```python
from build123d import *

# Parameters (mm, degrees)
SKETCH1_R              = 21.209
EXTRUDE1_DEPTH         = 63.5
SKETCH2_R              = 17.78
EXTRUDE2_DEPTH         = 25.4
EXTRUDE2_DRAFT         = -2.87
CIRPATTERN1_COUNT      = 12
CHAMFER2_SIZE          = 0.254
CHAMFER2_SIZE2         = 0.267741651
CHAMFER2_EDGE_2_SIZE   = 0.254
CHAMFER2_EDGE_2_SIZE2  = 0.267741651
CHAMFER2_EDGE_3_SIZE   = 0.254
CHAMFER2_EDGE_3_SIZE2  = 0.267741651
CHAMFER2_EDGE_4_SIZE   = 0.254
CHAMFER2_EDGE_4_SIZE2  = 0.267741651
CHAMFER2_EDGE_5_SIZE   = 0.254
CHAMFER2_EDGE_5_SIZE2  = 0.267741651
CHAMFER2_EDGE_6_SIZE   = 0.254
CHAMFER2_EDGE_6_SIZE2  = 0.267741651
CHAMFER2_EDGE_7_SIZE   = 0.254
CHAMFER2_EDGE_7_SIZE2  = 0.267741651
CHAMFER2_EDGE_8_SIZE   = 0.254
CHAMFER2_EDGE_8_SIZE2  = 0.267741651
CHAMFER2_EDGE_9_SIZE   = 0.254
CHAMFER2_EDGE_9_SIZE2  = 0.267741651
CHAMFER2_EDGE_10_SIZE  = 0.254
CHAMFER2_EDGE_10_SIZE2 = 0.267741651
CHAMFER2_EDGE_11_SIZE  = 0.254
CHAMFER2_EDGE_11_SIZE2 = 0.267741651
CHAMFER2_EDGE_12_SIZE  = 0.254
CHAMFER2_EDGE_12_SIZE2 = 0.267741651


with BuildPart() as part:
    # Sketch1 → Extrude1 (new body)
    with BuildSketch(Plane(origin=(0, 0, 0), x_dir=(0, 0, -1), z_dir=(1, 0, 0))):
        Circle(SKETCH1_R)
    extrude(amount=EXTRUDE1_DEPTH)


with BuildPart() as extrude2_tool:
    # Sketch2 → Extrude2 (with draft: the straight prism first)
    with BuildSketch(Plane(origin=(63.5, 0, 0), x_dir=(0, 0, -1), z_dir=(1, 0, 0))):
        Circle(SKETCH2_R)
    extrude(amount=-EXTRUDE2_DEPTH)
    # Extrude2: the draft: its side faces are tilted about the plane it starts from
    extrude2_sides = [extrude2_tool.faces().sort_by_distance(p)[0] for p in [
        (50.8, 0, 17.78),
    ]]
    draft(extrude2_sides, Plane(origin=(63.5, 0, 0), x_dir=(0, 0, -1), z_dir=(1, 0, 0)), EXTRUDE2_DRAFT)


with BuildPart() as part_1:
    add(part.part)

    # Extrude2: cut by extrude2_tool
    add(extrude2_tool.part, mode=Mode.SUBTRACT)

    # Sketch4 → 3/16 (0.1875) Diameter Hole1 (revolve, cut)
    with BuildSketch(Plane(origin=(63.5, 0, 16.51), x_dir=(0, 0, -1), z_dir=(0, 1, 0))):
        Polygon((0, 0), (0, 33.180799349), (2.38125, 31.75), (2.38125, 0), align=None)
    f_3_16_0_1875_diameter_hole1 = revolve(axis=Axis((69.85, 0, 16.51), (-1, 0, 0)), mode=Mode.SUBTRACT)

    # CirPattern1: 3/16 (0.1875) Diameter Hole1 ×12 about axis
    cirpattern1_axis = Axis((0, 0, 0), (1, 0, 0))
    for i in range(1, CIRPATTERN1_COUNT):
        add(f_3_16_0_1875_diameter_hole1.rotate(cirpattern1_axis, i * 360 / CIRPATTERN1_COUNT), mode=Mode.SUBTRACT)

    # Chamfer2
    chamfer2_edges = [part_1.edges().sort_by_distance(p)[0] for p in [
        (63.5, 17.174161191, -4.601802622),
    ]]
    chamfer2_side = [part_1.faces().sort_by_distance(p)[0] for p in [
        (63.5, 0, 20.609118891),
    ]]
    chamfer(chamfer2_edges, length=CHAMFER2_SIZE, length2=CHAMFER2_SIZE2, reference=chamfer2_side[0])

    # Chamfer2 edge 2
    chamfer2_edge_2_edges = [part_1.edges().sort_by_distance(p)[0] for p in [
        (63.5, 12.572358569, -12.572358569),
    ]]
    chamfer2_edge_2_side = [part_1.faces().sort_by_distance(p)[0] for p in [
        (63.5, 0, 20.609118891),
    ]]
    chamfer(chamfer2_edge_2_edges, length=CHAMFER2_EDGE_2_SIZE, length2=CHAMFER2_EDGE_2_SIZE2, reference=chamfer2_edge_2_side[0])

    # Chamfer2 edge 3
    chamfer2_edge_3_edges = [part_1.edges().sort_by_distance(p)[0] for p in [
        (63.5, 4.601802622, -17.174161191),
    ]]
    chamfer2_edge_3_side = [part_1.faces().sort_by_distance(p)[0] for p in [
        (63.5, 0, 20.609118891),
    ]]
    chamfer(chamfer2_edge_3_edges, length=CHAMFER2_EDGE_3_SIZE, length2=CHAMFER2_EDGE_3_SIZE2, reference=chamfer2_edge_3_side[0])

    # Chamfer2 edge 4
    chamfer2_edge_4_edges = [part_1.edges().sort_by_distance(p)[0] for p in [
        (63.5, -4.601802622, -17.174161191),
    ]]
    chamfer2_edge_4_side = [part_1.faces().sort_by_distance(p)[0] for p in [
        (63.5, 0, 20.609118891),
    ]]
    chamfer(chamfer2_edge_4_edges, length=CHAMFER2_EDGE_4_SIZE, length2=CHAMFER2_EDGE_4_SIZE2, reference=chamfer2_edge_4_side[0])

    # Chamfer2 edge 5
    chamfer2_edge_5_edges = [part_1.edges().sort_by_distance(p)[0] for p in [
        (63.5, -12.572358569, -12.572358569),
    ]]
    chamfer2_edge_5_side = [part_1.faces().sort_by_distance(p)[0] for p in [
        (63.5, 0, 20.609118891),
    ]]
    chamfer(chamfer2_edge_5_edges, length=CHAMFER2_EDGE_5_SIZE, length2=CHAMFER2_EDGE_5_SIZE2, reference=chamfer2_edge_5_side[0])

    # Chamfer2 edge 6
    chamfer2_edge_6_edges = [part_1.edges().sort_by_distance(p)[0] for p in [
        (63.5, -17.174161191, -4.601802622),
    ]]
    chamfer2_edge_6_side = [part_1.faces().sort_by_distance(p)[0] for p in [
        (63.5, 0, 20.609118891),
    ]]
    chamfer(chamfer2_edge_6_edges, length=CHAMFER2_EDGE_6_SIZE, length2=CHAMFER2_EDGE_6_SIZE2, reference=chamfer2_edge_6_side[0])

    # Chamfer2 edge 7
    chamfer2_edge_7_edges = [part_1.edges().sort_by_distance(p)[0] for p in [
        (63.5, -17.174161191, 4.601802622),
    ]]
    chamfer2_edge_7_side = [part_1.faces().sort_by_distance(p)[0] for p in [
        (63.5, 0, 20.609118891),
    ]]
    chamfer(chamfer2_edge_7_edges, length=CHAMFER2_EDGE_7_SIZE, length2=CHAMFER2_EDGE_7_SIZE2, reference=chamfer2_edge_7_side[0])

    # Chamfer2 edge 8
    chamfer2_edge_8_edges = [part_1.edges().sort_by_distance(p)[0] for p in [
        (63.5, -12.572358569, 12.572358569),
    ]]
    chamfer2_edge_8_side = [part_1.faces().sort_by_distance(p)[0] for p in [
        (63.5, 0, 20.609118891),
    ]]
    chamfer(chamfer2_edge_8_edges, length=CHAMFER2_EDGE_8_SIZE, length2=CHAMFER2_EDGE_8_SIZE2, reference=chamfer2_edge_8_side[0])

    # Chamfer2 edge 9
    chamfer2_edge_9_edges = [part_1.edges().sort_by_distance(p)[0] for p in [
        (63.5, -4.601802622, 17.174161191),
    ]]
    chamfer2_edge_9_side = [part_1.faces().sort_by_distance(p)[0] for p in [
        (63.5, 0, 20.609118891),
    ]]
    chamfer(chamfer2_edge_9_edges, length=CHAMFER2_EDGE_9_SIZE, length2=CHAMFER2_EDGE_9_SIZE2, reference=chamfer2_edge_9_side[0])

    # Chamfer2 edge 10
    chamfer2_edge_10_edges = [part_1.edges().sort_by_distance(p)[0] for p in [
        (63.5, 4.601802622, 17.174161191),
    ]]
    chamfer2_edge_10_side = [part_1.faces().sort_by_distance(p)[0] for p in [
        (63.5, 0, 20.609118891),
    ]]
    chamfer(chamfer2_edge_10_edges, length=CHAMFER2_EDGE_10_SIZE, length2=CHAMFER2_EDGE_10_SIZE2, reference=chamfer2_edge_10_side[0])

    # Chamfer2 edge 11
    chamfer2_edge_11_edges = [part_1.edges().sort_by_distance(p)[0] for p in [
        (63.5, 12.572358569, 12.572358569),
    ]]
    chamfer2_edge_11_side = [part_1.faces().sort_by_distance(p)[0] for p in [
        (63.5, 0, 20.609118891),
    ]]
    chamfer(chamfer2_edge_11_edges, length=CHAMFER2_EDGE_11_SIZE, length2=CHAMFER2_EDGE_11_SIZE2, reference=chamfer2_edge_11_side[0])

    # Chamfer2 edge 12
    chamfer2_edge_12_edges = [part_1.edges().sort_by_distance(p)[0] for p in [
        (63.5, 17.174161191, 4.601802622),
    ]]
    chamfer2_edge_12_side = [part_1.faces().sort_by_distance(p)[0] for p in [
        (63.5, 0, 20.609118891),
    ]]
    chamfer(chamfer2_edge_12_edges, length=CHAMFER2_EDGE_12_SIZE, length2=CHAMFER2_EDGE_12_SIZE2, reference=chamfer2_edge_12_side[0])


solid = part_1.part
```
Can you work these out from the model? Positions are in its coordinate system, mm. Give positions to 0.01 mm unless a question says otherwise; leave off trailing zeros. Order: outer loops, then holes, each group sorted by start corner. A loop starts at its lowest first (then second) coordinate and runs counter-clockwise, first axis right, second up. Notation, with made-up numbers: M 4,-4.75 L 17,-4.75 A28 ccw 17,29.25 Z; hole C -6,-8 d11. An arc over 180 degrees is marked long. One line per item, written item: value.
1) I want a section at A-A, the plane x = 44. List the corners of the cut face in (y, z) for me (1 decimal), plus the area to 3 significant figures.
Answer sheet:
outline: C 0,0 d42.4; hole M -16.6,-2.4 A16.8 ccw -15.6,-6.3 A2.4 ccw -13.2,-10.4 A16.8 ccw -10.4,-13.2 A2.4 ccw -6.3,-15.6 A16.8 ccw -2.4,-16.6 A2.4 ccw 2.4,-16.6 A16.8 ccw 6.3,-15.6 A2.4 ccw 10.4,-13.2 A16.8 ccw 13.2,-10.4 A2.4 ccw 15.6,-6.3 A16.8 ccw 16.6,-2.4 A2.4 ccw 16.6,2.4 A16.8 ccw 15.6,6.3 A2.4 ccw 13.2,10.4 A16.8 ccw 10.4,13.2 A2.4 ccw 6.3,15.6 A16.8 ccw 2.4,16.6 A2.4 ccw -2.4,16.6 A16.8 ccw -6.3,15.6 A2.4 ccw -10.4,13.2 A16.8 ccw -13.2,10.4 A2.4 ccw -15.6,6.3 A16.8 ccw -16.6,2.4 A2.4 ccw Z
area: 433 mm^2
2) I want a section at B-B, the plane x = 17. List the corners of the cut face in (y, z) for me, plus the area to 3 significant figures.
Answer sheet:
outline: C 0,0 d42.42
area: 1,410 mm^2
3) Please list where these lines run through material, in increasing order: line 1 along Y through (x, z) = (38, 15); line 2 along X through (y, z) = (-0.5, 7.5); line 3 along Z through (x, y) = (60.5, 7).
Answer sheet:
line 1: y = -14.99 to -10.53, -5.98 to -1.84, 1.84 to 5.98, 10.53 to 14.99
line 2: x = 0 to 38.1
line 3: z = -20.02 to -16.32, 16.32 to 20.02
4) We'd pull the mould along X, two halves only. Please class faces 1 (the face through (31.31, 6.37, -20.23)), 2 (the face through (0, 0, 0)), 3 (the face through (50.842, -12.099, 12.148)): released by +X, released by -X, zero draft, split by the parting line, or undercut.
Answer sheet:
face 1: zero draft
face 2: released by -X
face 3: released by +X
5) For P1, Ø4, axis at x = 53, y = 8.5, coming from the +Z side; P2, Ø16.5, axis at y = -3.5, z = 6.5, coming from the +X side; P3, Ø4.5, axis at y = -14.3, z = -8.25, coming from the +X side, each with a flat end and sliding along its axis, tell me the tip position at first contact or that it passes through.
Answer sheet:
P1: stops at z = 20.19
P2: stops at x = 38.1
P3: stops at x = 31.67
6) I want a section at C-C, the plane x = 55.5. List the corners of the cut face in (y, z) for me (1 decimal), plus the area to 3 significant figures.
Answer sheet:
outline: C 0,0 d42.4; hole M -17.2,-2.3 A17.4 ccw -16.1,-6.6 A2.4 ccw -13.8,-10.6 A17.4 ccw -10.6,-13.8 A2.4 ccw -6.6,-16.1 A17.4 ccw -2.3,-17.2 A2.4 ccw 2.3,-17.2 A17.4 ccw 6.6,-16.1 A2.4 ccw 10.6,-13.8 A17.4 ccw 13.8,-10.6 A2.4 ccw 16.1,-6.6 A17.4 ccw 17.2,-2.3 A2.4 ccw 17.2,2.3 A17.4 ccw 16.1,6.6 A2.4 ccw 13.8,10.6 A17.4 ccw 10.6,13.8 A2.4 ccw 6.6,16.1 A17.4 ccw 2.3,17.2 A2.4 ccw -2.3,17.2 A17.4 ccw -6.6,16.1 A2.4 ccw -10.6,13.8 A17.4 ccw -13.8,10.6 A2.4 ccw -16.1,6.6 A17.4 ccw -17.2,2.3 A2.4 ccw Z
area: 403 mm^2
